Could you check a few things on this drawing? It's one solid part, dimensions in mm from its lowest x, y, z. A direction names the side the tool comes from. Round coordinates to 2 decimals unless told otherwise and drop trailing zeros. Loops run counter-clockwise (first coordinate to the right, second up) from the corner with the lowest first, then second, coordinate; pieces in that order, holes last. Notation, with made-up numbers: M 70.5,-16.75 L 92.5,-16.75 A17 ccw 92.5,9.25 Z; hole C -10.5,-9.75 d3. An arc over 180 degrees is marked long. Write item = value, one per line. Start each with the question number.
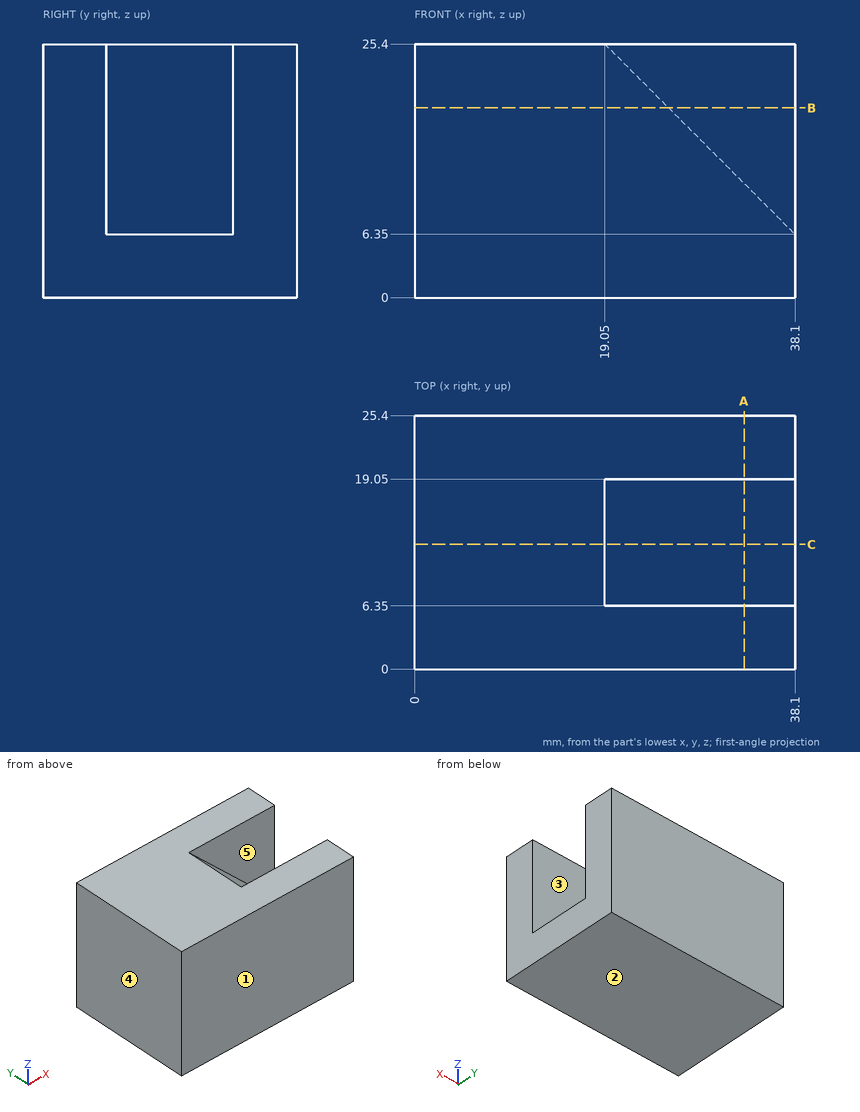
Item 1: Please list where these lines run through material, in increasing order: line 1 (Z direction, x = 25, y = 8); line 2 (Z direction, x = 26, y = 11); line 3 (X direction, y = 14, z = 12.25). Write a range as [from, to].
Item 2: We'd pull the mould along Y, two halves only. Please class the marked faces 1, 2 and 3: released by +Y, released by -Y, zero draft, split by the parting line, or undercut.
Item 3: I want a section at C-C, the plane y = 12.5. List the corners of the cut face in (x, z) for me.
Item 4: For the marked faces 4 and 5, which set-ups out of +Z, -Z, +X, -X, +Y, -Y let a thin tool reach every point of the face, with its end or its side?
Item 5: I want a section at B-B, the plane z = 19. List the corners of the cut face in (x, y) for me.
Item 6: I want a section at A-A, the plane x = 33. List the corners of the cut face in (y, z) for me, then the cut area to 3 significant figures.
Item 7: Will this pin go through, and if not, where does the flat tip stop? pin 1 Ø1 at (y, z) = (18, 16.5) entering from +X.
Worked out:
q1.line_1 = [0, 19.45]
q1.line_2 = [0, 18.45]
q1.line_3 = [0, 32.2]
q2.face_1 = released by -Y
q2.face_2 = zero draft
q2.face_3 = undercut
q3.outline = M 0,0 L 38.1,0 L 38.1,6.35 L 19.05,25.4 L 0,25.4 Z
q4.face_4 = +Z, -Z, -X, +Y, -Y
q4.face_5 = +Z, +X
q5.outline = M 0,0 L 38.1,0 L 38.1,6.35 L 25.45,6.35 L 25.45,19.05 L 38.1,19.05 L 38.1,25.4 L 0,25.4 Z
q6.outline = M 0,0 L 25.4,0 L 25.4,25.4 L 19.05,25.4 L 19.05,11.45 L 6.35,11.45 L 6.35,25.4 L 0,25.4 Z
q6.area = 468 mm2
q7.pin_1 = 28.45
